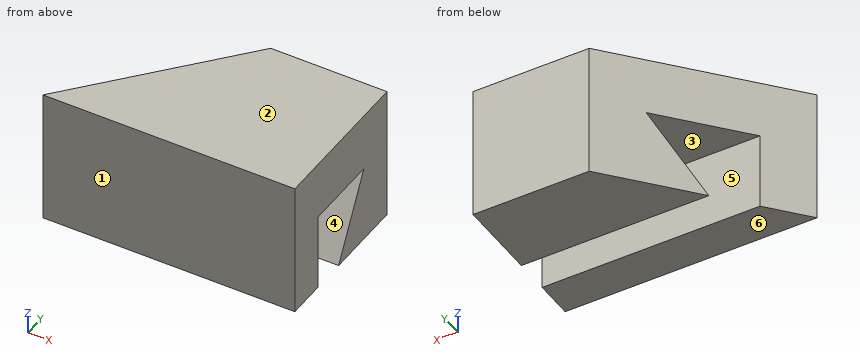
```python
from build123d import *

# Parameters (mm, degrees)
BOSS_EXTRU_1_DEPTH = 65
CHANFREIN1_SIZE2   = 40
CHANFREIN1_SIZE    = 35


with BuildPart() as part:
    # Esquisse1 → Boss.-Extru.1 (new body)
    with BuildSketch(Plane(origin=(0, 0, 0), x_dir=(0, 0, -1), z_dir=(1, 0, 0))):
        Polygon((-21.204724929, -24.063055062), (13.795275071, -24.063055062), (13.795275071, -14.063055062), (-6.204724929, -14.063055062), (-6.204724929, 5.936944938), (13.795275071, -5.063055062), (13.795275071, 15.936944938), (-21.204724929, 15.936944938), align=None)
    extrude(amount=BOSS_EXTRU_1_DEPTH)

    # Chanfrein1
    chanfrein1_edges = [part.edges().sort_by_distance(p)[0] for p in [
        (0, 15.936944938, 3.704724929),
    ]]
    chanfrein1_side = [part.faces().sort_by_distance(p)[0] for p in [
        (0.7, 15.936944938, 3.704724929),
    ]]
    chamfer(chanfrein1_edges, length=CHANFREIN1_SIZE - 0.0001, length2=CHANFREIN1_SIZE2 - 0.0001, reference=chanfrein1_side[0])  # a hair under: the kernel refuses the full size


solid = part.part
```
Design review of the part built by this model. Coordinates are the model's own, in mm. Face numbers are marked on the shaded views. A direction names the side the tool comes from. Give positions to 0.01 mm unless a question says otherwise; leave off trailing zeros. Write each loop counter-clockwise with the first axis right and the second up, starting at its lowest first coordinate (ties: lowest second). Pieces come first, ordered by that corner, then holes.
(1) Add section A-A (y = -3). Give the boundary of the cut face in (x, z).
Checked values:
outline: (18.43, -13.8) - (65, -13.8) - (65, -10.04) - (18.43, -10.04) - close; (18.43, 6.2) - (65, 6.2) - (65, 21.2) - (18.43, 21.2) - close
(2) Tool access review of the marked faces 4, 5 and 6: name each direction out of +Z, -Z, +X, -X, +Y, -Y from which nothing blocks a thin tool from reaching the whole face with its end or side.
Checked values:
face 4: +X, -X
face 5: -Z, +X, -X
face 6: -Z, +X, -X, +Y, -Y
(3) Clearance check with flat-ended pins moving along their axes: pin 1 Ø4 at (y, z) = (-5.5, 5.5) entering from -X; pin 2 Ø1.5 at (x, z) = (10.5, 14.5) entering from +Y; pin 3 Ø5 at (y, z) = (3, -9.5) entering from -X; pin 4 Ø2 at (x, y) = (11.5, -8.5) entering from -Z. State where each tip first meets the part, or that it passes through.
Checked values:
pin 1: stops at x = 14.6
pin 2: stops at y = -11.21
pin 3: stops at x = 21.49
pin 4: passes through
(4) Add section C-C (x = 46). Give the boundary of the cut face in (y, z).
Checked values:
outline: (-24.06, -13.8) - (-14.06, -13.8) - (-14.06, 6.2) - (5.94, 6.2) - (-5.06, -13.8) - (15.94, -13.8) - (15.94, 21.2) - (-24.06, 21.2) - close
(5) Wall thickness on line 1 along Y through (x, z) = (55, 1.5); line 2 along Z through (x, y) = (59, 0); line 3 along Y through (x, z) = (51, -9.5): over which ranges is each line inside the solid? List them lowest first.
Checked values:
line 1: y = -24.06 to -14.06, 3.35 to 15.94
line 2: z = -13.8 to -4.59, 6.2 to 21.2
line 3: y = -24.06 to -14.06, -2.7 to 15.94
(6) Mouldability with a two-part tool opening along Y and no side actions: class the marked faces 1, 2 and 3 as +Y half, -Y half, draft (parallel to the pull), parting line (faces both ways), or undercut.
Checked values:
face 1: -Y half
face 2: draft
face 3: undercut
